from build123d import *

# Parameters (mm, degrees)
SKETCH1_R           = 4.5
BOSS_EXTRUDE1_DEPTH = 10
CUT_EXTRUDE1_DEPTH  = 3
SKETCH3_R           = 2.75
SKETCH3_R_2         = 1.75
BOSS_EXTRUDE2_DEPTH = 1.5
CHAMFER1_SIZE       = 1


with BuildPart() as part:
    # Sketch1 → Boss-Extrude1 (new body)
    with BuildSketch(Plane(origin=(0, 0, 0), x_dir=(1, 0, 0), z_dir=(0, 1, 0))):
        Circle(SKETCH1_R)
    extrude(amount=BOSS_EXTRUDE1_DEPTH)

    # Sketch2 → Cut-Extrude1 (cut)
    with BuildSketch(Plane.XZ):
        with BuildLine():
            Line((-1, 1.05), (1, 1.05))
            ThreePointArc((1, 1.05), (0, -1.45), (-1, 1.05))
        make_face()
    extrude(amount=-CUT_EXTRUDE1_DEPTH, mode=Mode.SUBTRACT)

    # Sketch3 → Boss-Extrude2 (add)
    with BuildSketch(Plane.XZ):
        Circle(SKETCH3_R)
        Circle(SKETCH3_R_2, mode=Mode.SUBTRACT)
    extrude(amount=BOSS_EXTRUDE2_DEPTH)

    # Chamfer1
    chamfer1_edges = [part.edges().sort_by_distance(p)[0] for p in [
        (-4.5, 0, 0),
    ]]
    chamfer(chamfer1_edges, length=CHAMFER1_SIZE)


solid = part.part
Check sheet for the modelled part. Datum: model origin and axes. Units: mm. A direction names the side the tool comes from. Round coordinates to 2 decimals unless told otherwise and drop trailing zeros. Loops run counter-clockwise (first coordinate to the right, second up) from the corner with the lowest first, then second, coordinate; pieces in that order, holes last. Notation, with made-up numbers: (-2, 75.5) -> (52, 75.5) arc R16 ccw to (52, 100.5) -> close; hole circle Ø6 at (-14.5, 59). An arc over 180 degrees is marked (long way). Put each result on its own line as item: value. Start each with the question number.
1. Draft check along Z on faces 3 (the face through (-0.596, -0.74, -2.685)), 4 (the face through (0, 1, 1.05)), 5 (the face through (0, 10, 0)). Enter one of: +Z half, -Z half, draft (parallel to the pull), parting line (faces both ways), or undercut.
2. Section check B-B (z = 0). Enter the section's corners in (x, y), plus the area to 3 significant figures.
3. Scan lines: probe 1 along Z at (x, y) = (0, -1.05); probe 2 along Z at (x, y) = (0, 1.5); probe 3 along Y at (x, z) = (-1.5, 0). Record each from-to range of solid material in increasing order.
4. Section check A-A (x = 0). Enter the section's corners in (y, z).
5. Gauge pin test, flat ends, axial feed: pin 1 (2 mm diameter, centred on x = -1, y = 6.5, fed in from +Z); pin 2 (5 mm diameter, centred on y = 0, z = -3, fed in from +X); pin 3 (1.5 mm diameter, centred on y = 8.5, z = 3, fed in from -X); pin 4 (3 mm diameter, centred on x = 0, z = 0, fed in from -Y). Record the tip position at first contact, or that the pin passes through.
6. Access from +Z, -Z, +X, -X, +Y, -Y to the whole of each face (thin tool, end or side, straight path). Record for faces 1 (the face through (-0.4, 0, 1.3)), 2 (the face through (-0.59, 5.44, -4.46)).
7. Section check D-D (y = 2.75). Enter the section's corners in (x, z), plus the area to 3 significant figures.
8. Section check C-C (y = 5.25). Enter the section's corners in (x, z).
Findings:
1. face 3: parting line
1. face 4: undercut
1. face 5: draft
2. outline: (-4.5, 1) -> (-3.5, 0) -> (-2.75, 0) -> (-2.75, -1.5) -> (-1.75, -1.5) -> (-1.75, 0) -> (-1.45, 0) -> (-1.45, 3) -> (1.45, 3) -> (1.45, 0) -> (1.75, 0) -> (1.75, -1.5) -> (2.75, -1.5) -> (2.75, 0) -> (3.5, 0) -> (4.5, 1) -> (4.5, 10) -> (-4.5, 10) -> close
2. area: 83.3 mm^2
3. probe 1: z = -2.75 to -1.75, 1.75 to 2.75
3. probe 2: z = -4.5 to -1.45, 1.05 to 4.5
3. probe 3: y = 0 to 10
4. outline: (-1.5, -2.75) -> (0, -2.75) -> (0, -3.5) -> (1, -4.5) -> (10, -4.5) -> (10, 4.5) -> (1, 4.5) -> (0, 3.5) -> (0, 2.75) -> (-1.5, 2.75) -> (-1.5, 1.75) -> (0, 1.75) -> (0, 1.05) -> (3, 1.05) -> (3, -1.45) -> (0, -1.45) -> (0, -1.75) -> (-1.5, -1.75) -> close
5. pin 1: stops at z = 4.5
5. pin 2: stops at x = 4.44
5. pin 3: stops at x = -3.9
5. pin 4: stops at y = 0
6. face 1: -Y
6. face 2: +Y, -Y
7. outline: circle Ø9 at (0, 0); hole (-1, 1.05) arc R1.45 ccw (long way) to (1, 1.05) -> close
7. area: 57.6 mm^2
8. outline: circle Ø9 at (0, 0)
